from build123d import *

# Parameters (mm, degrees)
SKETCH3_R          = 2.5
CUT_EXTRUDE1_DEPTH = 10


with BuildPart() as part:
    # Sketch2 → Revolve1 (revolve)
    with BuildSketch(Plane.XY, mode=Mode.PRIVATE) as revolve1_sk:
        with BuildLine():
            Line((0, 0), (10, 0))
            Line((10, 0), (10, 0.216117819))
            ThreePointArc((10, 0.216117819), (9.923207143, 0.41656375), (9.732142857, 0.514390909))
            ThreePointArc((9.732142857, 0.514390909), (7.5, 3), (9.732142857, 5.485609091))
            ThreePointArc((9.732142857, 5.485609091), (9.923207143, 5.58343625), (10, 5.783882181))
            Line((10, 5.783882181), (10, 6))
            Line((10, 6), (0, 6))
            Line((0, 6), (0, 0))
        make_face()
    revolve(revolve1_sk.sketch.rotate(Axis((0, 0, 0), (0, 1, 0)), 90), axis=Axis((0, 0, 0), (0, 1, 0)))

    # Sketch3 → Cut-Extrude1 (cut)
    with BuildSketch(Plane(origin=(0, 6, 0), x_dir=(1, 0, 0), z_dir=(0, 1, 0))):
        with Locations(Location((0, 0, 0), (0, 0, 270))):
            Circle(SKETCH3_R)
    extrude(amount=-CUT_EXTRUDE1_DEPTH, mode=Mode.SUBTRACT)


solid = part.part
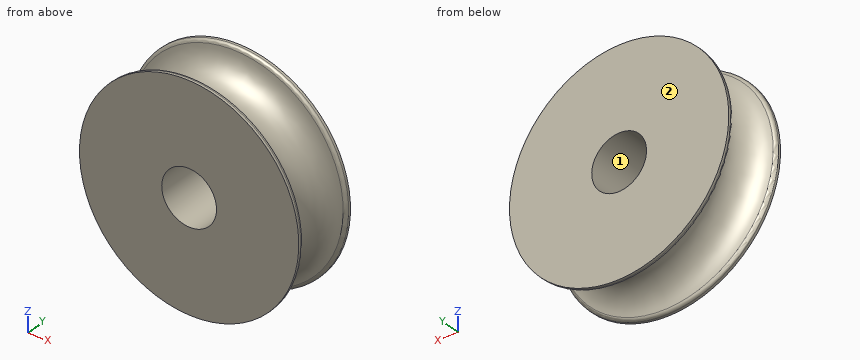
CAD build for the part. Positions are in the model's coordinates, mm. Face numbers are marked on the shaded views. Coordinates: 2 decimals unless noted, no trailing zeros. Loops run counter-clockwise (first coordinate to the right, second up) from the corner with the lowest first, then second, coordinate; pieces in that order, holes last. Notation, with made-up numbers: (79, 81.5) -> (104, 81.5) arc R5 cw to (104, 87.5) -> close; hole circle Ø8 at (17, 42). An arc over 180 degrees is marked (long way). One line per item, written item: value.
1. Slice it at A-A on x = 0. Write the cut outline in (y, z), and give its area (3 significant figures).
Answers:
outline: (0, -10) -> (0.22, -10) arc R0.3 ccw to (0.51, -9.73) arc R2.5 cw to (5.49, -9.73) arc R0.3 ccw to (5.78, -10) -> (6, -10) -> (6, -2.5) -> (0, -2.5) -> close; (0, 2.5) -> (6, 2.5) -> (6, 10) -> (5.78, 10) arc R0.3 ccw to (5.49, 9.73) arc R2.5 cw to (0.51, 9.73) arc R0.3 ccw to (0.22, 10) -> (0, 10) -> close
area: 70.3 mm^2
2. Slice it at D-D on y = 2.2. Write the cut outline in (x, z), and give its area (3 significant figures).
Answers:
outline: circle Ø15.26 at (0, 0); hole circle Ø5 at (0, 0)
area: 163 mm^2
3. Pull direction Z, two halves, no side cores. Call the marked faces 1 and 2: pulls with the +Z half, pulls with the -Z half, needs draft (parallel to the pull), parting line crosses it, or undercut.
Answers:
face 1: undercut
face 2: needs draft
4. Drill centre lines: line 1 (Y direction, x = -1, z = 8.75); line 2 (X direction, y = 1.9, z = 0) (3 decimals); line 3 (X direction, y = 3.3, z = -1.5). Where is each one in solid material? Low to high. Write a range as [from, to].
Answers:
line 1: y = [0, 0.8], [5.2, 6]
line 2: x = [-7.755, -2.5], [2.5, 7.755]
line 3: x = [-7.37, -2], [2, 7.37]
5. Slice it at C-C on y = 4.45. Write the cut outline in (x, z), and give its area (3 significant figures).
Answers:
outline: circle Ø15.93 at (0, 0); hole circle Ø5 at (0, 0)
area: 180 mm^2
6. Flat gauge pins, fed straight in: P1, Ø2, axis at x = 1, y = 1, coming from the -Z side; P2, Ø2, axis at y = 5.5, z = -3, coming from the -X side. Where does each tip first touch, or does it go through?
Answers:
P1: stops at z = -9.99
P2: stops at x = -9.79
7. Slice it at B-B on z = 0. Write the cut outline in (x, y), and give its area (3 significant figures).
Answers:
outline: (-10, 0) -> (-2.5, 0) -> (-2.5, 6) -> (-10, 6) -> (-10, 5.78) arc R0.3 ccw to (-9.73, 5.49) arc R2.5 cw to (-9.73, 0.51) arc R0.3 ccw to (-10, 0.22) -> close; (2.5, 0) -> (10, 0) -> (10, 0.22) arc R0.3 ccw to (9.73, 0.51) arc R2.5 cw to (9.73, 5.49) arc R0.3 ccw to (10, 5.78) -> (10, 6) -> (2.5, 6) -> close
area: 70.3 mm^2
